from build123d import *

# Parameters (mm, degrees)
SKETCH1_R             = 30
SKETCH1_R_2           = 2
BOSS_EXTRUDE1_DEPTH   = 6
M3X0_5_TAPPED_HOLE1_D = 2.5
CHAMFER1_SIZE         = 1
BOSS_EXTRUDE2_DEPTH   = 1


with BuildPart() as part:
    # Sketch1 → Boss-Extrude1 (new body)
    with BuildSketch(Plane(origin=(0, 0, 0), x_dir=(1, 0, 0), z_dir=(0, 1, 0))):
        with Locations(Location((0, 0, 0), (0, 0, 270))):
            Circle(SKETCH1_R)
        with Locations(Location((0, 0, 0), (0, 0, 270))):
            Circle(SKETCH1_R_2, mode=Mode.SUBTRACT)
        with BuildLine():
            Line((-22.449944321, -3), (-13.610657589, -3))
            ThreePointArc((-13.610657589, -3), (-12.465954646, -3.359983179), (-11.733325508, -4.310344828))
            ThreePointArc((-11.733325508, -4.310344828), (-8.838834765, -8.838834765), (-4.310344828, -11.733325508))
            ThreePointArc((-4.310344828, -11.733325508), (-3.359983179, -12.465954646), (-3, -13.610657589))
            Line((-3, -13.610657589), (-3, -22.449944321))
            ThreePointArc((-3, -22.449944321), (-3.748913516, -24.010323316), (-5.434782609, -24.402113392))
            ThreePointArc((-5.434782609, -24.402113392), (-17.67766953, -17.67766953), (-24.402113392, -5.434782609))
            ThreePointArc((-24.402113392, -5.434782609), (-24.010323316, -3.748913516), (-22.449944321, -3))
        make_face(mode=Mode.SUBTRACT)
        with BuildLine():
            Line((3, -22.449944321), (3, -13.610657589))
            ThreePointArc((3, -13.610657589), (3.359983179, -12.465954646), (4.310344828, -11.733325508))
            ThreePointArc((4.310344828, -11.733325508), (8.838834765, -8.838834765), (11.733325508, -4.310344828))
            ThreePointArc((11.733325508, -4.310344828), (12.465954646, -3.359983179), (13.610657589, -3))
            Line((13.610657589, -3), (22.449944321, -3))
            ThreePointArc((22.449944321, -3), (24.010323316, -3.748913516), (24.402113392, -5.434782609))
            ThreePointArc((24.402113392, -5.434782609), (17.67766953, -17.67766953), (5.434782609, -24.402113392))
            ThreePointArc((5.434782609, -24.402113392), (3.748913516, -24.010323316), (3, -22.449944321))
        make_face(mode=Mode.SUBTRACT)
        with BuildLine():
            Line((22.449944321, 3), (13.610657589, 3))
            ThreePointArc((13.610657589, 3), (12.465954646, 3.359983179), (11.733325508, 4.310344828))
            ThreePointArc((11.733325508, 4.310344828), (8.838834765, 8.838834765), (4.310344828, 11.733325508))
            ThreePointArc((4.310344828, 11.733325508), (3.359983179, 12.465954646), (3, 13.610657589))
            Line((3, 13.610657589), (3, 22.449944321))
            ThreePointArc((3, 22.449944321), (3.748913516, 24.010323316), (5.434782609, 24.402113392))
            ThreePointArc((5.434782609, 24.402113392), (17.67766953, 17.67766953), (24.402113392, 5.434782609))
            ThreePointArc((24.402113392, 5.434782609), (24.010323316, 3.748913516), (22.449944321, 3))
        make_face(mode=Mode.SUBTRACT)
        with BuildLine():
            Line((-3, 22.449944321), (-3, 13.610657589))
            ThreePointArc((-3, 13.610657589), (-3.359983179, 12.465954646), (-4.310344828, 11.733325508))
            ThreePointArc((-4.310344828, 11.733325508), (-8.838834765, 8.838834765), (-11.733325508, 4.310344828))
            ThreePointArc((-11.733325508, 4.310344828), (-12.465954646, 3.359983179), (-13.610657589, 3))
            Line((-13.610657589, 3), (-22.449944321, 3))
            ThreePointArc((-22.449944321, 3), (-24.010323316, 3.748913516), (-24.402113392, 5.434782609))
            ThreePointArc((-24.402113392, 5.434782609), (-17.67766953, 17.67766953), (-5.434782609, 24.402113392))
            ThreePointArc((-5.434782609, 24.402113392), (-3.748913516, 24.010323316), (-3, 22.449944321))
        make_face(mode=Mode.SUBTRACT)
    extrude(amount=BOSS_EXTRUDE1_DEPTH)

    # M3x0.5 Tapped Hole1 (through all)
    with Locations(Plane(origin=(0, 6, 0), x_dir=(1, 0, 0), z_dir=(0, 1, 0))):
        with Locations((-7.361215932, -4.25), (0, 8.5), (7.361215932, -4.25)):
            Hole(M3X0_5_TAPPED_HOLE1_D / 2)

    # Sketch5 → Cut-Revolve1 (revolve, cut)
    with BuildSketch(Plane(origin=(0, 0, 0), x_dir=(0, 0, -1), z_dir=(1, 0, 0)), mode=Mode.PRIVATE) as cut_revolve1_sk:
        with BuildLine():
            Line((-30, 4.5), (-27, 4.5))
            ThreePointArc((-27, 4.5), (-25.5, 3), (-27, 1.5))
            Line((-27, 1.5), (-30, 1.5))
            Line((-30, 1.5), (-30, 4.5))
        make_face()
    revolve(cut_revolve1_sk.sketch.rotate(Axis((0, 0, 0), (0, 1, 0)), 180), axis=Axis((0, 0, 0), (0, 1, 0)), mode=Mode.SUBTRACT)

    # Chamfer1
    chamfer1_edges = [part.edges().sort_by_distance(p)[0] for p in [
        (0, 4.5, -30),
        (0, 1.5, -30),
        (-12.465954646, 0, 3.359983179),
        (-18.030300955, 0, 3),
        (-24.010323316, 0, 3.748913516),
        (-17.67766953, 0, 17.67766953),
        (-3.748913516, 0, 24.010323316),
        (-3, 0, 18.030300955),
        (-3.359983179, 0, 12.465954646),
        (-8.838834765, 0, 8.838834765),
        (-12.465954646, 6, 3.359983179),
        (-18.030300955, 6, 3),
        (-24.010323316, 6, 3.748913516),
        (-17.67766953, 6, 17.67766953),
        (-3.748913516, 6, 24.010323316),
        (-3, 6, 18.030300955),
        (-3.359983179, 6, 12.465954646),
        (-8.838834765, 6, 8.838834765),
        (24.010323316, 0, 3.748913516),
        (18.030300955, 0, 3),
        (12.465954646, 0, 3.359983179),
        (8.838834765, 0, 8.838834765),
        (3.359983179, 0, 12.465954646),
        (3, 0, 18.030300955),
        (3.748913516, 0, 24.010323316),
        (17.67766953, 0, 17.67766953),
        (24.010323316, 6, 3.748913516),
        (18.030300955, 6, 3),
        (12.465954646, 6, 3.359983179),
        (8.838834765, 6, 8.838834765),
        (3.359983179, 6, 12.465954646),
        (3, 6, 18.030300955),
        (3.748913516, 6, 24.010323316),
        (17.67766953, 6, 17.67766953),
        (17.67766953, 0, -17.67766953),
        (3.748913516, 0, -24.010323316),
        (3, 0, -18.030300955),
        (3.359983179, 0, -12.465954646),
        (8.838834765, 0, -8.838834765),
        (12.465954646, 0, -3.359983179),
        (18.030300955, 0, -3),
        (24.010323316, 0, -3.748913516),
        (17.67766953, 6, -17.67766953),
        (3.748913516, 6, -24.010323316),
        (3, 6, -18.030300955),
        (3.359983179, 6, -12.465954646),
        (8.838834765, 6, -8.838834765),
        (12.465954646, 6, -3.359983179),
        (18.030300955, 6, -3),
        (24.010323316, 6, -3.748913516),
        (-24.010323316, 0, -3.748913516),
        (-18.030300955, 0, -3),
        (-12.465954646, 0, -3.359983179),
        (-8.838834765, 0, -8.838834765),
        (-3.359983179, 0, -12.465954646),
        (-3, 0, -18.030300955),
        (-3.748913516, 0, -24.010323316),
        (-17.67766953, 0, -17.67766953),
        (-24.010323316, 6, -3.748913516),
        (-18.030300955, 6, -3),
        (-12.465954646, 6, -3.359983179),
        (-8.838834765, 6, -8.838834765),
        (-3.359983179, 6, -12.465954646),
        (-3, 6, -18.030300955),
        (-3.748913516, 6, -24.010323316),
        (-17.67766953, 6, -17.67766953),
    ]]
    chamfer(chamfer1_edges, length=CHAMFER1_SIZE)

    # Sketch6 → Boss-Extrude2 (add)
    with BuildSketch(Plane(origin=(0, 6, 0), x_dir=(1, 0, 0), z_dir=(0, 1, 0))):
        Polygon((24, -1.5), (24, 1.5), (28, 0), align=None)
    extrude(amount=BOSS_EXTRUDE2_DEPTH)


solid = part.part
The model under review builds one solid part; all positions refer to its coordinate system, in mm. Round coordinates to 2 decimals unless told otherwise and drop trailing zeros. Loops run counter-clockwise (first coordinate to the right, second up) from the corner with the lowest first, then second, coordinate; pieces in that order, holes last. Notation, with made-up numbers: M 5,43 L 36,43 A29 ccw 36,71 Z; hole C 75,-10.5 d5. An arc over 180 degrees is marked long. Answer as CSV lines item,"result". Start each with the question number.
Item 1: Insertion check: P1, Ø6.5, axis at x = 0, z = 0, coming from the +Y side; P2, Ø1.2, axis at y = 3, z = -17.5, coming from the -X side; P3, Ø1.5, axis at y = 6, z = 3, coming from the -X side. Each pin has a flat end and moves straight along its axis. Give the tip position at first contact, or say it passes through.
Item 2: Wall thickness on line 1 (Y direction, x = 25.5, z = -11.5); line 2 (X direction, y = 4, z = 17); line 3 (Z direction, x = -9, y = 4): over which ranges is each line inside the solid? List them lowest first. Write a range as [from, to].
Item 3: Consider section A-A (x = 0). Write out the cut boundary in (y, z), then the cut area to 3 significant figures.
Item 4: Consider section B-B (z = -8.5). State how many separate pieces and enclosed holes the cut face has, then the cut area to 3 significant figures.
Item 5: Mouldability with a two-part tool opening along X and no side actions: class faces 1 (the face through (-17.537, 2.972, 17.817)), 2 (the face through (8.79, 2.97, 8.89)), 3 (the face through (0, 6, 6)), 4 (the face through (26.03, 6.49, 0.74)) as released by +X, released by -X, zero draft, split by the parting line, or undercut.
Answer:
1,P1,"stops at y = 6"
1,P2,"stops at x = -19.1"
1,P3,"stops at x = -29.92"
2,line 1,"y = [0, 1.5], [4.5, 6]"
2,line 2,"x = [-19.52, -18.33], [-3, 3], [18.33, 19.52]"
2,line 3,"z = [-24.27, -23.32], [-8.67, 8.67], [23.32, 24.27]"
3,outline,"M 0,-30 L 0.5,-30 L 1.5,-29 L 1.5,-27 A1.5 cw 4.5,-27 L 4.5,-29 L 5.5,-30 L 6,-30 L 6,-9.75 L 0,-9.75 Z; M 0,-7.25 L 6,-7.25 L 6,-2 L 0,-2 Z; M 0,2 L 6,2 L 6,30 L 5.5,30 L 4.5,29 L 4.5,27 A1.5 cw 1.5,27 L 1.5,29 L 0.5,30 L 0,30 Z"
3,area,"294 mm^2"
4,separate pieces,"4"
4,enclosed holes,"0"
4,area,"125 mm^2"
5,face 1,"undercut"
5,face 2,"undercut"
5,face 3,"zero draft"
5,face 4,"released by +X"
